Check sheet for the modelled part. Datum: model origin and axes. Units: mm. Coordinates: 2 decimals unless noted, no trailing zeros. Loops run counter-clockwise (first coordinate to the right, second up) from the corner with the lowest first, then second, coordinate; pieces in that order, holes last. Notation, with made-up numbers: (-20.75, -0.75) - (2.25, -0.75) arc R13 cw to (2.25, 19.25) - close; hole circle Ø7 at (34, 46.25). An arc over 180 degrees is marked (long way). Use a Markdown table: item, result. Add a question column.
1) Thickness scan on line 1 (Z direction, x = 1, y = -0.6); line 2 (Z direction, x = -7.25, y = -2.5); line 3 (X direction, y = -3.6, z = -13). Record the ranges inside material, lowest first.
2) Sectioned sample at C-C, the plane y = -1.5. Enter the section's corners in (x, z), then the cut area to 3 significant figures.
3) Sectioned sample at A-A, the plane z = -4.5. Enter the section's corners in (x, y), then the cut area to 3 significant figures.
4) Draft check along Z on faces 1 (the flat face through (-2, -3, -18.382)), 2 (the cylindrical face through (0.612, -2.616, -7.223)), 3 (the flat face through (-2, 0, -9)), 4 (the cylindrical face through (-5.836, -2.616, -14.984)). Enter one of: pulls with the +Z half, pulls with the -Z half, needs draft (parallel to the pull), parting line crosses it, or undercut.
5) Sectioned sample at B-B, the plane x = 1.5. Enter the section's corners in (y, z), then the cut area to 3 significant figures.
from build123d import *

# Parameters (mm, degrees)
F0_W     = 15.9
F0_H     = 18.6
F1_DEPTH = 5.16
F2_R     = 2.45
F3_DEPTH = 5.161
F4_R     = 2.44
F5_DEPTH = 5.161


with BuildPart() as f1:
    # F0 (on Front) → F1 (new body)
    with BuildSketch(Plane.XZ):
        with Locations((-1.597295, -9.081725)):
            Rectangle(F0_W, F0_H)
    extrude(amount=F1_DEPTH)

    # F2 (on face) → F3 (cut, through all)
    with BuildSketch(Plane.XZ.offset(5.16)):
        with Locations((1.142705, -4.831725)):
            Circle(F2_R)
    extrude(amount=-F3_DEPTH, mode=Mode.SUBTRACT)

    # F4 (on face) → F5 (cut, through all)
    with BuildSketch(Plane.XZ.offset(5.16)):
        with Locations((-5.307295, -12.601725)):
            Circle(F4_R)
    extrude(amount=-F5_DEPTH, mode=Mode.SUBTRACT)


solid = f1.part
Solved:
| question | item | result |
|---|---|---|
| 1 | line 1 | z = -18.38 to -7.28, -2.39 to 0.22 |
| 1 | line 2 | z = -18.38 to -14.08, -11.13 to 0.22 |
| 1 | line 3 | x = -9.55 to -7.71, -2.9 to 6.35 |
| 2 | outline | (-9.55, -18.38) - (6.35, -18.38) - (6.35, 0.22) - (-9.55, 0.22) - close; hole circle Ø4.88 at (-5.31, -12.6); hole circle Ø4.9 at (1.14, -4.83) |
| 2 | area | 258 mm2 |
| 3 | outline | (-9.55, -5.16) - (-1.28, -5.16) - (-1.28, 0) - (-9.55, 0) - close; (3.57, -5.16) - (6.35, -5.16) - (6.35, 0) - (3.57, 0) - close |
| 3 | area | 57.0 mm2 |
| 4 | face 1 | pulls with the -Z half |
| 4 | face 2 | undercut |
| 4 | face 3 | needs draft |
| 4 | face 4 | undercut |
| 5 | outline | (-5.16, -18.38) - (0, -18.38) - (0, -7.26) - (-5.16, -7.26) - close; (-5.16, -2.41) - (0, -2.41) - (0, 0.22) - (-5.16, 0.22) - close |
| 5 | area | 71.0 mm2 |
